Input: part model. Units: mm. Frame: model coordinates. Round coordinates to 2 decimals unless told otherwise and drop trailing zeros. Loops run counter-clockwise (first coordinate to the right, second up) from the corner with the lowest first, then second, coordinate; pieces in that order, holes last. Notation, with made-up numbers: (56, 69.25) - (75, 69.25) arc R28 cw to (75, 103.25) - close; hole circle Ø11 at (64, 72.25). An arc over 180 degrees is marked (long way). One line per question, with ' | ' between items. Start each with the question number.
Item 1: Section B-B, the plane z = -8.5. Return loops of the section in (x, y), plus the area to 3 significant figures.
Item 2: Draft query along X for faces 1 (the face through (5.12, 0.25, -8.87)), 2 (the face through (17.33, 0.25, -10.48)), 3 (the face through (57, 0, -11)). Return one class per face: pulls with the +X half, pulls with the -X half, needs draft (parallel to the pull), parting line crosses it, or undercut.
Item 3: Section A-A, the plane x = 76. Return loops of the section in (y, z).
Item 4: Material intervals for line 1 along X through (y, z) = (0.4, -10.25); line 2 along X through (y, z) = (0.2, -9); line 3 along Y through (x, z) = (91.5, -1), sorted ascending.
Item 5: Section C-C, the plane z = -14.75. Return loops of the section in (x, y).
```python
from build123d import *

# Parameters (mm, degrees)
EXTRUDE_1_DEPTH     = 0.5
SKETCH_2_R          = 2.75
CUT_EXTRUDE_1_DEPTH = 10
CHAMFER_1_SIZE      = 3
CHAMFER_1_SIZE2     = 0.209780436
CHAMFER_2_SIZE      = 0.2
CHAMFER_2_SIZE2     = 2.860133251


with BuildPart() as part:
    # 草图1 → 凸台-拉伸1 (new body)
    with BuildSketch(Plane(origin=(0, 0, 0), x_dir=(1, 0, 0), z_dir=(0, 1, 0))):
        Polygon((0, 0), (10.392304845, 18), (110.392304845, 18), (100, 0), align=None)
    extrude(amount=EXTRUDE_1_DEPTH)

    # 草图2 → 切除-拉伸1 (cut)
    with BuildSketch(Plane(origin=(0, 0, 0), x_dir=(-1, 0, 0), z_dir=(0, -1, 0))):
        with Locations(Location((-15.011106999, 9, 0), (0, 0, 90))):
            Circle(SKETCH_2_R)
    extrude(amount=-CUT_EXTRUDE_1_DEPTH, mode=Mode.SUBTRACT)

    # 倒角1
    chamfer_1_edges = [part.edges().sort_by_distance(p)[0] for p in [
        (50, 0, 0),
    ]]
    chamfer_1_side = [part.faces().sort_by_distance(p)[0] for p in [
        (55.733651423, 0, -9),
    ]]
    chamfer(chamfer_1_edges, length=CHAMFER_1_SIZE, length2=CHAMFER_1_SIZE2, reference=chamfer_1_side[0])

    # 倒角2
    chamfer_2_edges = [part.edges().sort_by_distance(p)[0] for p in [
        (50, 0.5, 0),
    ]]
    chamfer_2_side = [part.faces().sort_by_distance(p)[0] for p in [
        (50, 0.354890218, 0),
    ]]
    chamfer(chamfer_2_edges, length=CHAMFER_2_SIZE, length2=CHAMFER_2_SIZE2, reference=chamfer_2_side[0])


solid = part.part
```
Return value:
1) outline: (4.91, 0) - (12.31, 0) - (12.31, 0.5) - (4.91, 0.5) - close; (17.72, 0) - (104.91, 0) - (104.91, 0.5) - (17.72, 0.5) - close | area: 47.3 mm2
2) face 1: pulls with the -X half | face 2: undercut | face 3: needs draft
3) outline: (0, -18) - (0.5, -18) - (0.5, -2.86) - (0.3, 0) - (0.21, 0) - (0, -3) - close
4) line 1: 5.92 to 12.56, 17.46 to 105.92 | line 2: 5.2 to 12.26, 17.76 to 105.2 | line 3: 0.14 to 0.37
5) outline: (8.52, 0) - (108.52, 0) - (108.52, 0.5) - (8.52, 0.5) - close
